Verification items for the finished model (mm, model axes). A direction names the side the tool comes from. Give positions to 0.01 mm unless a question says otherwise; leave off trailing zeros. Use CSV: the item, a comma, the result in double quotes.
from build123d import *

# Parameters (mm, degrees)
CROQUIS1_R              = 1.5875
CROQUIS1_W              = 2.3
CROQUIS1_H              = 5
SALIENTE_EXTRUIR1_DEPTH = 3.5


with BuildPart() as part:
    # Croquis1 → Saliente-Extruir1 (new body)
    with BuildSketch(Plane(origin=(0, 0, 0), x_dir=(1, 0, 0), z_dir=(0, 1, 0))):
        with BuildLine():
            Line((-15.874295221, 31.874668373), (-11.754060701, 36.031005585))
            ThreePointArc((-11.754060701, 36.031005585), (-10.369805081, 36.191711772), (-9.114574915, 35.586412398))
            Line((-9.114574915, 35.586412398), (-2.716116368, 29.839829039))
            ThreePointArc((-2.716116368, 29.839829039), (-1.851993104, 29.164348948), (-0.781901657, 28.923752474))
            Line((-0.781901657, 28.923752474), (0.565649151, 28.923752474))
            Line((0.565649151, 28.923752474), (0.647095514, 28.923752474))
            Line((0.647095514, 28.923752474), (1.994646322, 28.923752474))
            ThreePointArc((1.994646322, 28.923752474), (3.06473777, 29.164348948), (3.928861034, 29.839829039))
            Line((3.928861034, 29.839829039), (10.327319581, 35.586412398))
            ThreePointArc((10.327319581, 35.586412398), (11.582549747, 36.191711772), (12.966805367, 36.031005585))
            Line((12.966805367, 36.031005585), (17.087039886, 31.874668373))
            ThreePointArc((17.087039886, 31.874668373), (17.703192062, 31.303268278), (18.365142407, 30.785616548))
            ThreePointArc((18.365142407, 30.785616548), (19.626123842, 28.369336027), (18.427544181, 25.921501773))
            ThreePointArc((18.427544181, 25.921501773), (16.902388008, 24.495249114), (15.706675307, 22.783358599))
            add(Edge.make_bspline(
                [(17.08637633, -26.708053998), (12.010093305, -21.41999504), (5.252678849, -14.724182661), (6.940083791, 4.589437635), (12.242427811, 16.518318459), (15.706675307, 22.783358599)],
                knots=[0, 0, 0, 0, 0.308743397, 0.525126437, 0.93919625, 0.93919625, 0.93919625, 0.93919625], degree=3))
            ThreePointArc((17.08637633, -26.708053998), (19.60196336, -29.831990985), (16.763044461, -32.665310574))
            ThreePointArc((16.763044461, -32.665310574), (15.724835901, -32.951926252), (14.903555585, -33.648721922))
            ThreePointArc((14.903555585, -33.648721922), (13.755521453, -34.435837646), (12.364591814, -34.382468459))
            Line((12.364591814, -34.382468459), (9.205112275, -34.382468459))
            ThreePointArc((9.205112275, -34.382468459), (8.113093326, -34.633581042), (7.240450136, -35.336472768))
            Line((7.240450136, -35.336472768), (6.559598907, -36.201703273))
            ThreePointArc((6.559598907, -36.201703273), (5.686955717, -36.904594998), (4.594936767, -37.155707581))
            Line((4.594936767, -37.155707581), (4.047588743, -37.155707581))
            Line((4.047588743, -37.155707581), (2.140229158, -31.696312325))
            ThreePointArc((2.140229158, -31.696312325), (1.548523338, -30.753735958), (0.606372333, -30.161353086))
            ThreePointArc((0.606372333, -30.161353086), (-0.335778672, -30.753735958), (-0.927484492, -31.696312325))
            Line((-0.927484492, -31.696312325), (-2.834844078, -37.155707581))
            Line((-2.834844078, -37.155707581), (-3.382192102, -37.155707581))
            ThreePointArc((-3.382192102, -37.155707581), (-4.474211051, -36.904594998), (-5.346854241, -36.201703273))
            Line((-5.346854241, -36.201703273), (-6.02770547, -35.336472768))
            ThreePointArc((-6.02770547, -35.336472768), (-6.90034866, -34.633581042), (-7.99236761, -34.382468459))
            Line((-7.99236761, -34.382468459), (-11.151847148, -34.382468459))
            ThreePointArc((-11.151847148, -34.382468459), (-12.542776787, -34.435837646), (-13.690810919, -33.648721922))
            ThreePointArc((-13.690810919, -33.648721922), (-14.512091235, -32.951926252), (-15.550299796, -32.665310574))
            ThreePointArc((-15.550299796, -32.665310574), (-18.389218694, -29.831990985), (-15.873631664, -26.708053998))
            add(Edge.make_bspline(
                [(-15.873631664, -26.708053998), (-10.797348639, -21.41999504), (-4.039934183, -14.724182661), (-5.727339125, 4.589437635), (-11.029683145, 16.518318459), (-14.493930641, 22.783358599)],
                knots=[0, 0, 0, 0, 0.308743397, 0.525126437, 0.93919625, 0.93919625, 0.93919625, 0.93919625], degree=3))
            ThreePointArc((-14.493930641, 22.783358599), (-15.689643342, 24.495249114), (-17.214799516, 25.921501773))
            ThreePointArc((-17.214799516, 25.921501773), (-18.413379177, 28.369336027), (-17.152397742, 30.785616548))
            ThreePointArc((-17.152397742, 30.785616548), (-16.490447396, 31.303268278), (-15.874295221, 31.874668373))
        make_face()
        with Locations(Location((16.606372333, -29.669404393, 0), (0, 0, 270))):
            Circle(CROQUIS1_R, mode=Mode.SUBTRACT)
        with Locations(Location((-15.393627667, 28.330595607, 0), (0, 0, 270))):
            Circle(CROQUIS1_R, mode=Mode.SUBTRACT)
        with Locations(Location((16.606372333, 28.330595607, 0), (0, 0, 270))):
            Circle(CROQUIS1_R, mode=Mode.SUBTRACT)
        with Locations(Location((-15.393627667, -29.669404393, 0), (0, 0, 270))):
            Circle(CROQUIS1_R, mode=Mode.SUBTRACT)
        with BuildLine():
            Line((-3.287471504, -24.301852689), (-3.287471504, -31.696312325))
            ThreePointArc((-3.287471504, -31.696312325), (-4.722504291, -33.131345111), (-6.157537077, -31.696312325))
            Line((-6.157537077, -31.696312325), (-6.157537077, -24.301852689))
            ThreePointArc((-6.157537077, -24.301852689), (-4.722504291, -22.866819903), (-3.287471504, -24.301852689))
        make_face(mode=Mode.SUBTRACT)
        with BuildLine():
            Line((-0.787449287, -21.665575324), (2.000193952, -21.665575324))
            ThreePointArc((2.000193952, -21.665575324), (2.783225968, -21.287556725), (2.974256652, -20.439297049))
            Line((2.974256652, -20.439297049), (1.580435032, -14.439297049))
            ThreePointArc((1.580435032, -14.439297049), (0.606372333, -13.665575324), (-0.367690367, -14.439297049))
            Line((-0.367690367, -14.439297049), (-1.761511986, -20.439297049))
            ThreePointArc((-1.761511986, -20.439297049), (-1.570481302, -21.287556725), (-0.787449287, -21.665575324))
        make_face(mode=Mode.SUBTRACT)
        with BuildLine():
            Line((4.50021617, -24.301852689), (4.50021617, -31.696312325))
            ThreePointArc((4.50021617, -31.696312325), (5.935248956, -33.131345111), (7.370281743, -31.696312325))
            Line((7.370281743, -31.696312325), (7.370281743, -24.301852689))
            ThreePointArc((7.370281743, -24.301852689), (5.935248956, -22.866819903), (4.50021617, -24.301852689))
        make_face(mode=Mode.SUBTRACT)
        with BuildLine():
            Line((-0.39543432, 25.732977828), (1.608178986, 25.732977828))
            ThreePointArc((1.608178986, 25.732977828), (3.877356766, 24.695331568), (4.576798655, 22.300199296))
            Line((4.576798655, 22.300199296), (3.080222057, 12.034517445))
            ThreePointArc((3.080222057, 12.034517445), (0.606372333, 9.895166222), (-1.867477392, 12.034517445))
            Line((-1.867477392, 12.034517445), (-3.364053989, 22.300199296))
            ThreePointArc((-3.364053989, 22.300199296), (-2.6646121, 24.695331568), (-0.39543432, 25.732977828))
        make_face(mode=Mode.SUBTRACT)
        with Locations((-10.043627667, 27.05538099)):
            Rectangle(CROQUIS1_W, CROQUIS1_H, mode=Mode.SUBTRACT)
        with Locations((11.256372333, 27.05538099)):
            Rectangle(CROQUIS1_W, CROQUIS1_H, mode=Mode.SUBTRACT)
    extrude(amount=SALIENTE_EXTRUIR1_DEPTH)


solid = part.part
(1) Tool access check on faces 1 (the flat face through (4.5, 2, 28)), 2 (the flat face through (11, 2, 34.382)), 3 (the cylindrical face through (3.051, 1.726, -29.158)). Record the directions out of +Z, -Z, +X, -X, +Y, -Y that give a thin tool (end or side, any length) a straight path to the whole face; none if there is none.
Calculated:
face 1,"+Y, -Y"
face 2,"+Z, +Y, -Y"
face 3,"-Z, +Y, -Y"
(2) Section check A-A on y = 1.25. Count the separate pieces of the cut face and the enclosed holes in it, plus the area to 3 significant figures.
Calculated:
separate pieces,"1"
enclosed holes,"10"
area,"1,290 mm²"
(3) Mould release check, pull along X, two halves, no side actions. Record for faces 4 (the flat face through (1, 3.5, 0)), 5 (the cylindrical face through (3.854, 1.726, -24.722)), 6 (the flat face through (-13.843, 1.726, -33.924)): released by +X, released by -X, zero draft, split by the parting line, or undercut.
Calculated:
face 4,"zero draft"
face 5,"undercut"
face 6,"released by -X"
(4) Scan lines: L1, parallel to X at y = 1.85, z = 27; L2, parallel to X at y = 0.25, z = 32; L3, parallel to Z at x = 11, y = 3.1. Record each from-to range of solid material in increasing order. Write a range as from..to.
Calculated:
L1,"x = -16.76..-6.16, -3.29..4.5, 7.37..17.98"
L2,"x = -17.28..-6.13, -3.32..-1.03, 2.25..4.53, 7.34..18.5"
L3,"z = -36.02..-29.56, -24.56..-13.03, 20.08..34.38"
(5) Depth check by flat-ended pin: pin 1 Ø1.8 at (x, y) = (-9.5, 2.5) entering from +Z; pin 2 Ø2 at (x, y) = (1, 1) entering from +Z; pin 3 Ø8 at (x, z) = (13, 8) entering from -Y; pin 4 Ø2 at (x, y) = (0, 2.5) entering from -Z. Enter the tip coordinate at first touch or a pass-through.
Calculated:
pin 1,"stops at z = 34.38"
pin 2,"stops at z = 31.37"
pin 3,"passes through"
pin 4,"stops at z = -28.93"
